Source: CAD feature listing. Evaluate the final solid. Frame: model axes, mm. Face numbers are marked on the shaded views. Coordinates: 2 decimals unless noted, no trailing zeros. Order: outer loops, then holes, each group sorted by start corner. A loop starts at its lowest first (then second) coordinate and runs counter-clockwise, first axis right, second up. Notation, with made-up numbers: (79, 20.25) -> (125, 20.25) arc R12 cw to (125, 31.25) -> close; hole circle Ø3 at (50.25, 11). An arc over 180 degrees is marked (long way). Put each result on its own line as item: value.
from build123d import *

# Parameters (mm, degrees)
F0_W           = 38.1
F0_H           = 38.1
F1_DEPTH       = 8.255
F2_R           = 5.08
F3_D           = 8.4328
F3_CBORE_D     = 15.24
F3_CBORE_DEPTH = 5.08


with BuildPart() as f1:
    # F0 (on Top) → F1 (new body)
    with BuildSketch(Plane.XY):
        Rectangle(F0_W, F0_H)
    extrude(amount=-F1_DEPTH)

    # F2
    f2_edges = [f1.edges().sort_by_distance(p)[0] for p in [
        (-19.05, 19.05, -4.1275),
        (-19.05, -19.05, -4.1275),
        (19.05, -19.05, -4.1275),
        (19.05, 19.05, -4.1275),
    ]]
    fillet(f2_edges, radius=F2_R)

    # F3 (through all)
    with Locations(Plane.XY):
        with Locations((0, 0)):
            CounterBoreHole(F3_D / 2, F3_CBORE_D / 2, F3_CBORE_DEPTH)


solid = f1.part
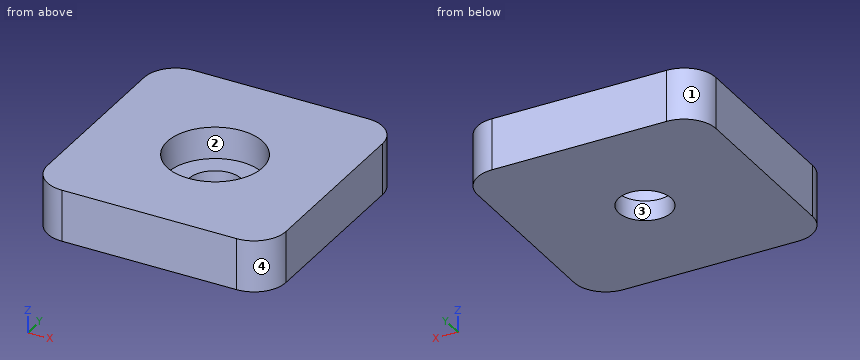
1. Cut plane B-B on x = 0. Output: boundary loops of the cut face in (y, z) (3 decimals).
Numbers:
outline: (-19.05, -8.255) -> (-4.216, -8.255) -> (-4.216, -5.08) -> (-7.62, -5.08) -> (-7.62, 0) -> (-19.05, 0) -> close; (4.216, -8.255) -> (19.05, -8.255) -> (19.05, 0) -> (7.62, 0) -> (7.62, -5.08) -> (4.216, -5.08) -> close
2. Cut plane D-D on z = -6.75. Output: boundary loops of the cut face in (x, y), plus the area to 3 significant figures.
Numbers:
outline: (-19.05, -13.97) arc R5.08 ccw to (-13.97, -19.05) -> (13.97, -19.05) arc R5.08 ccw to (19.05, -13.97) -> (19.05, 13.97) arc R5.08 ccw to (13.97, 19.05) -> (-13.97, 19.05) arc R5.08 ccw to (-19.05, 13.97) -> close; hole circle Ø8.43 at (0, 0)
area: 1,370 mm2
3. Cut plane A-A on z = -2.5. Output: boundary loops of the cut face in (x, y).
Numbers:
outline: (-19.05, -13.97) arc R5.08 ccw to (-13.97, -19.05) -> (13.97, -19.05) arc R5.08 ccw to (19.05, -13.97) -> (19.05, 13.97) arc R5.08 ccw to (13.97, 19.05) -> (-13.97, 19.05) arc R5.08 ccw to (-19.05, 13.97) -> close; hole circle Ø15.24 at (0, 0)
4. Ray query, line 1 along Y through (x, z) = (0, -7.45); line 2 along Y through (x, z) = (0, -2.85); line 3 along X through (y, z) = (4.5, -3). Return the intervals inside material, ascending.
Numbers:
line 1: y = -19.05 to -4.22, 4.22 to 19.05
line 2: y = -19.05 to -7.62, 7.62 to 19.05
line 3: x = -19.05 to -6.15, 6.15 to 19.05
5. Pull-direction query (X, two-part tool) for the marked faces 1, 2, 3 and 4; classes: pulls with the +X half, pulls with the -X half, needs draft (parallel to the pull), parting line crosses it, or undercut.
Numbers:
face 1: pulls with the -X half
face 2: undercut
face 3: undercut
face 4: pulls with the +X half
